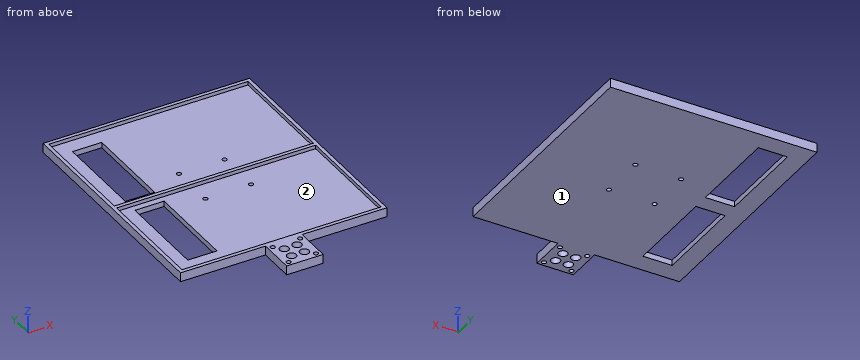
from build123d import *

# Parameters (mm, degrees)
F0_W      = 20
F0_H      = 20
F1_DEPTH  = 5
F3_D      = 2.5
F4_D      = 5
F5_W      = 109
F5_H      = 62
F6_DEPTH  = 2
F8_D      = 2.5
F9_W      = 16
F9_H      = 50
F10_DEPTH = 5.001


with BuildPart() as f1:
    # F0 (on Top) → F1 (new body)
    with BuildSketch(Plane.XY):
        Polygon((56.5, -65), (56.5, 65), (-56.5, 65), (-56.5, -65), (-10, -65), (-10, -45), (10, -45), (10, -65), align=None)
        with Locations((0, -75)):
            Rectangle(F0_W, F0_H)
        with Locations((0, -55)):
            Rectangle(F0_W, F0_H)
    extrude(amount=F1_DEPTH)

    # F3 (through all)
    with Locations(Plane.XY.offset(5)):
        with Locations((-7.5, -82.5), (-7.5, -67.5), (7.5, -67.5), (7.5, -82.5)):
            Hole(F3_D / 2)

    # F4 (through all)
    with Locations(Plane.XY.offset(5)):
        with Locations((-3.5, -71.5), (3.5, -71.5), (3.5, -78.5), (-3.5, -78.5)):
            Hole(F4_D / 2)

    # F5 (on face) → F6 (cut)
    with BuildSketch(Plane.XY.offset(5)):
        with Locations((0, 32)):
            Rectangle(F5_W, F5_H)
        with Locations((0, -32)):
            Rectangle(F5_W, F5_H)
    extrude(amount=-F6_DEPTH, mode=Mode.SUBTRACT)

    # F8 (through all)
    with Locations(Plane(origin=(0, 0, 0), x_dir=(1, 0, 0), z_dir=(0, 0, -1))):
        with Locations((-12.5, 12.5), (12.5, 12.5), (12.5, -12.5), (-12.5, -12.5)):
            Hole(F8_D / 2)

    # F9 (on face) → F10 (cut, through all)
    with BuildSketch(Plane(origin=(0, 0, 0), x_dir=(1, 0, 0), z_dir=(0, 0, -1))):
        with Locations((-38.4313402772, 29.4842413627)):
            Rectangle(F9_W, F9_H)
        with Locations((-38.4313402772, -29.4842413627)):
            Rectangle(F9_W, F9_H)
    extrude(amount=-F10_DEPTH, mode=Mode.SUBTRACT)


solid = f1.part
CAD build for the part. Positions are in the model's coordinates, mm. Face numbers are marked on the shaded views. Round coordinates to 2 decimals unless told otherwise and drop trailing zeros. Write each loop counter-clockwise with the first axis right and the second up, starting at its lowest first coordinate (ties: lowest second). Pieces come first, ordered by that corner, then holes. Notation, with made-up numbers: M -21,89 L 28,89 A23 ccw 28,100 Z; hole C 62,30.5 d6. An arc over 180 degrees is marked long. Put each result on its own line as item: value. Start each with the question number.
1) Saw through at A-A, the plane y = -71.5. Write the cut outline in (x, z).
2) Drill centre lines: probe 1 along Y at (x, z) = (-12.5, 1.2); probe 2 along X at (y, z) = (-82.5, 1.3); probe 3 along X at (y, z) = (12.5, 2.3). Where is each one in solid material? Low to high. Write a range as [from, to].
3) Saw through at C-C, the plane z = 0.95. Count the separate pieces of the cut face and the enclosed holes in it, and give its area (3 significant figures).
4) Saw through at D-D, the plane y = 39. Write the cut outline in (x, z), and give its area (3 significant figures).
5) Pull direction Y, two halves, no side cores. Call the marked faces 1 and 2: pulls with the +Y half, pulls with the -Y half, needs draft (parallel to the pull), parting line crosses it, or undercut.
6) Pin check, flat tips, straight feed: pin 1 Ø1.6 at (x, z) = (-13.5, 4) entering from -Y; pin 2 Ø3 at (x, y) = (12.5, 12.5) entering from +Z; pin 3 Ø1.5 at (y, z) = (-75.5, 1.5) entering from -X. Stop position of each tip, or through.
7) Saw through at B-B, the plane x = 3.5. Write the cut outline in (y, z).
Resolved:
1. outline: M -10,0 L -6,0 L -6,5 L -10,5 Z; M -1,0 L 1,0 L 1,5 L -1,5 Z; M 6,0 L 10,0 L 10,5 L 6,5 Z
2. probe 1: [-65, -13.75], [-11.25, 11.25], [13.75, 65]
2. probe 2: [-10, -8.75], [-6.25, 6.25], [8.75, 10]
2. probe 3: [-56.5, -46.43], [-30.43, -13.75], [-11.25, 11.25], [13.75, 56.5]
3. separate pieces: 1
3. enclosed holes: 14
3. area: 13,400 mm²
4. outline: M -56.5,0 L -46.43,0 L -46.43,3 L -54.5,3 L -54.5,5 L -56.5,5 Z; M -30.43,0 L 56.5,0 L 56.5,5 L 54.5,5 L 54.5,3 L -30.43,3 Z
4. area: 299 mm²
5. face 1: needs draft
5. face 2: undercut
6. pin 1: y = -65
6. pin 2: z = 3
6. pin 3: x = -10
7. outline: M -85,0 L -81,0 L -81,5 L -85,5 Z; M -76,0 L -74,0 L -74,5 L -76,5 Z; M -69,0 L 65,0 L 65,5 L 63,5 L 63,3 L 1,3 L 1,5 L -1,5 L -1,3 L -63,3 L -63,5 L -69,5 Z
